```python
from build123d import *

# Parameters (mm, degrees)
BOX013_W                   = 13.5
BOX013_H                   = 12.5
BOX013_DEPTH               = 2
BOX015001005_W             = 55
BOX015001005_H             = 4
BOX015001005_DEPTH         = 28
FILLET001_R                = 1
CYLINDER012029001024_R     = 1.5
CYLINDER012029001024_DEPTH = 6
CYLINDER012029001025_R     = 1.5
CYLINDER012029001025_DEPTH = 6
CYLINDER012029001026_R     = 1.5
CYLINDER012029001026_DEPTH = 6
CYLINDER012029001028_R     = 1.5
CYLINDER012029001028_DEPTH = 6
BOX015001024_W             = 5.5
BOX015001024_H             = 7
BOX015001024_DEPTH         = 2
BOX015001023_W             = 2.5
BOX015001023_H             = 12
BOX015001023_DEPTH         = 2
BOX015001022_W             = 5.5
BOX015001022_H             = 7
BOX015001022_DEPTH         = 2
CYLINDER012029001027_R     = 1.5
CYLINDER012029001027_DEPTH = 6
BOX015001025_W             = 2.5
BOX015001025_H             = 12
BOX015001025_DEPTH         = 2
BOX012_W                   = 304
BOX012_H                   = 50
BOX012_DEPTH               = 1.6


with BuildPart() as cube002:
    # Box013 → Box013 (new body)
    with BuildSketch(Plane(origin=(-37.4, 270.2, 11), x_dir=(1, 0, 0), z_dir=(0, -1, 0))):
        with Locations((6.75, 6.25)):
            Rectangle(BOX013_W, BOX013_H)
    extrude(amount=BOX013_DEPTH)


with BuildPart() as fillet001:
    # Box015001005 → Box015001005 (new body)
    with BuildSketch(Plane(origin=(-275.5, 267, 14), x_dir=(1, 0, 0), z_dir=(0, 0, 1))):
        with Locations((27.5, 2)):
            Rectangle(BOX015001005_W, BOX015001005_H)
    extrude(amount=BOX015001005_DEPTH)

    # Fillet001
    fillet001_edges = [fillet001.edges().sort_by_distance(p)[0] for p in [
        (-275.5, 269, 42),
        (-275.5, 269, 14),
        (-220.5, 269, 42),
        (-220.5, 269, 14),
    ]]
    fillet(fillet001_edges, radius=FILLET001_R)


with BuildPart() as cylinder012029001024:
    # Cylinder012029001024 → Cylinder012029001024 (new body)
    with BuildSketch(Plane(origin=(-248, 271, 8), x_dir=(1, 0, 0), z_dir=(0, -1, 0))):
        Circle(CYLINDER012029001024_R)
    extrude(amount=CYLINDER012029001024_DEPTH)


with BuildPart() as cylinder012029001025:
    # Cylinder012029001025 → Cylinder012029001025 (new body)
    with BuildSketch(Plane(origin=(-248, 271, 48), x_dir=(1, 0, 0), z_dir=(0, -1, 0))):
        Circle(CYLINDER012029001025_R)
    extrude(amount=CYLINDER012029001025_DEPTH)


with BuildPart() as cylinder012029001026:
    # Cylinder012029001026 → Cylinder012029001026 (new body)
    with BuildSketch(Plane(origin=(-288.5, 271, 17), x_dir=(1, 0, 0), z_dir=(0, -1, 0))):
        Circle(CYLINDER012029001026_R)
    extrude(amount=CYLINDER012029001026_DEPTH)


with BuildPart() as cylinder012029001028:
    # Cylinder012029001028 → Cylinder012029001028 (new body)
    with BuildSketch(Plane(origin=(-96.5, 271, 17), x_dir=(1, 0, 0), z_dir=(0, -1, 0))):
        Circle(CYLINDER012029001028_R)
    extrude(amount=CYLINDER012029001028_DEPTH)


with BuildPart() as cube021:
    # Box015001024 → Box015001024 (new body)
    with BuildSketch(Plane(origin=(-310, 270.2, 46), x_dir=(1, 0, 0), z_dir=(0, -1, 0))):
        with Locations((2.75, 3.5)):
            Rectangle(BOX015001024_W, BOX015001024_H)
    extrude(amount=BOX015001024_DEPTH)


with BuildPart() as cube020:
    # Box015001023 → Box015001023 (new body)
    with BuildSketch(Plane(origin=(-8.5, 270.2, 41), x_dir=(1, 0, 0), z_dir=(0, -1, 0))):
        with Locations((1.25, 6)):
            Rectangle(BOX015001023_W, BOX015001023_H)
    extrude(amount=BOX015001023_DEPTH)


with BuildPart() as cube019:
    # Box015001022 → Box015001022 (new body)
    with BuildSketch(Plane(origin=(-11.5, 270.2, 46), x_dir=(1, 0, 0), z_dir=(0, -1, 0))):
        with Locations((2.75, 3.5)):
            Rectangle(BOX015001022_W, BOX015001022_H)
    extrude(amount=BOX015001022_DEPTH)


with BuildPart() as cylinder012029001027:
    # Cylinder012029001027 → Cylinder012029001027 (new body)
    with BuildSketch(Plane(origin=(-207.5, 271, 17), x_dir=(1, 0, 0), z_dir=(0, -1, 0))):
        Circle(CYLINDER012029001027_R)
    extrude(amount=CYLINDER012029001027_DEPTH)


with BuildPart() as fusion001012:
    # Box015001025 → Box015001025 (new body)
    with BuildSketch(Plane(origin=(-310, 270.2, 41), x_dir=(1, 0, 0), z_dir=(0, -1, 0))):
        with Locations((1.25, 6)):
            Rectangle(BOX015001025_W, BOX015001025_H)
    extrude(amount=BOX015001025_DEPTH)

    # Fusion001012: union Cube002, Fillet001, Cylinder012029001024, Cylinder012029001025, Cylinder012029001026, Cylinder012029001028, Cube021, Cube020, Cube019, Cylinder012029001027
    add(cube002.part)
    add(fillet001.part)
    add(cylinder012029001024.part)
    add(cylinder012029001025.part)
    add(cylinder012029001026.part)
    add(cylinder012029001028.part)
    add(cube021.part)
    add(cube020.part)
    add(cube019.part)
    add(cylinder012029001027.part)


with BuildPart() as cut003025:
    # Box012 → Box012 (new body)
    with BuildSketch(Plane(origin=(-310, 270, 3), x_dir=(1, 0, 0), z_dir=(0, -1, 0))):
        with Locations((152, 25)):
            Rectangle(BOX012_W, BOX012_H)
    extrude(amount=BOX012_DEPTH)

    # Cut003025: cut Fusion001012
    add(fusion001012.part, mode=Mode.SUBTRACT)


solid = cut003025.part
```
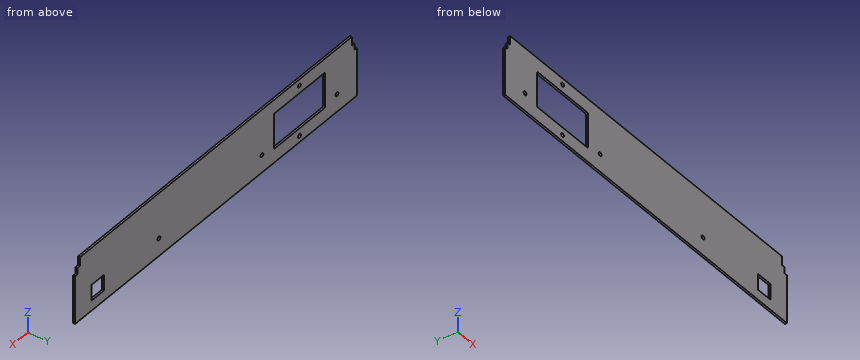
The listing builds one solid part. Answer for the finished solid, in the listing's coordinates (mm). Round coordinates to 2 decimals unless told otherwise and drop trailing zeros. Loops run counter-clockwise (first coordinate to the right, second up) from the corner with the lowest first, then second, coordinate; pieces in that order, holes last. Notation, with made-up numbers: (25, 79) - (34, 79) arc R37 ccw to (34, 115) - close; hole circle Ø11 at (50, 38). An arc over 180 degrees is marked (long way). Return JSON: item names as keys, results as strings. Group by question number.
1. Consider probe 1 along Z at (x, y) = (-248, 269.55); probe 2 along X at (y, z) = (269.4, 22); probe 3 along X at (y, z) = (269.5, 17). Determine where each line is inside the solid, lowest interval first.
2. The part is cut by section A-A on x = -34. Determine the outline of the cut face in (y, z), then the cut area to 3 significant figures.
3. Each of these flat-tipped pins is pushed along its axis until it touches: P1, Ø0.8, axis at x = -10.5, y = 269, coming from the +Z side; P2, Ø2.5, axis at x = -248, z = 8, coming from the +Y side; P3, Ø0.8, axis at y = 269, z = 50.5, coming from the +X side. Where does it stop, or does it pass through?
4. The part is cut by section C-C on y = 269.45. State how many separate pieces and enclosed holes the cut face has, then the cut area to 3 significant figures.
5. The part is cut by section B-B on z = 36. Determine the outline of the cut face in (x, y), then the cut area to 3 significant figures.
Resolved:
{
 "1": {"probe 1": "z = 3 to 6.5, 9.5 to 14, 42 to 46.5, 49.5 to 53", "probe 2": "x = -310 to -275.5, -220.5 to -37.4, -23.9 to -6", "probe 3": "x = -310 to -290, -287 to -275.5, -220.5 to -209, -206 to -98, -95 to -37.4, -23.9 to -6"},
 "2": {"outline": "(268.4, 3) - (270, 3) - (270, 11) - (268.4, 11) - close; (268.4, 23.5) - (270, 23.5) - (270, 53) - (268.4, 53) - close", "area": "60.0 mm²"},
 "3": {"P1": "stops at z = 46", "P2": "passes through", "P3": "stops at x = -11.5"},
 "4": {"separate pieces": "1", "enclosed holes": "7", "area": "13,400 mm²"},
 "5": {"outline": "(-310, 268.4) - (-275.5, 268.4) - (-275.5, 270) - (-310, 270) - close; (-220.5, 268.4) - (-6, 268.4) - (-6, 270) - (-220.5, 270) - close", "area": "398 mm²"}
}
